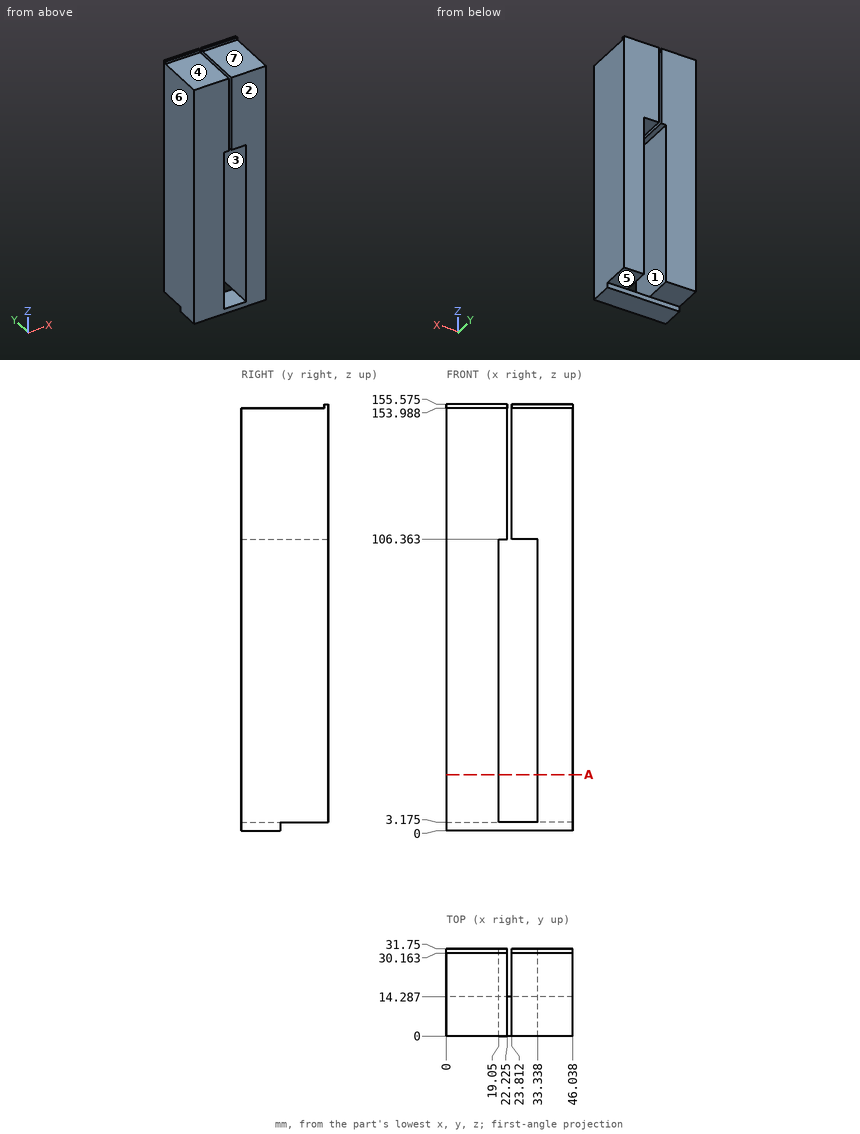
Job drawing, mm, ordinate dimensions from the low corner. One solid piece. A direction names the side the tool comes from. Round coordinates to 2 decimals unless told otherwise and drop trailing zeros. Write each loop counter-clockwise with the first axis right and the second up, starting at its lowest first coordinate (ties: lowest second). Pieces come first, ordered by that corner, then holes. Notation, with made-up numbers: (55, 5.25) -> (88, 5.25) arc R11 ccw to (88, 15.25) -> close; hole circle Ø6 at (76.5, 35). An arc over 180 degrees is marked (long way). Answer as a JSON object with one key per item and string values.
(1) Band-saw the part on A-A, the plane z = 20.5. List the corners of the cut face in (x, y).
Reported:
{"outline": "(0, 0) -> (19.05, 0) -> (19.05, 31.75) -> (0, 31.75) -> close; (33.34, 0) -> (46.04, 0) -> (46.04, 31.75) -> (33.34, 31.75) -> close"}
(2) Pin check, flat tips, straight feed: P1, Ø11, axis at x = 34.5, y = 20, coming from the +Z side; P2, Ø0.5, axis at x = 11, z = 155, coming from the -Y side; P3, Ø1.5, axis at x = 12.5, y = 22.5, coming from the -Z side (1 decimal). Stop position of each tip, or through.
Reported:
{"P1": "stops at z = 153.99", "P2": "stops at y = 30.16", "P3": "stops at z = 3.2"}
(3) Which spindle directions (+Z, -Z, +X, -X, +Y, -Y) get a long thin tool onto all of the face, cutting with end or side? Do the marked faces 5, 6 and 7. Say none if no direction does.
Reported:
{"face 5": "-Z, +X, -X, +Y", "face 6": "+Z, -Z, -X, +Y, -Y", "face 7": "+Z, +X, -X, -Y"}
(4) Probe probe 1 along X at (y, z) = (13, 66.5); probe 2 along Z at (x, y) = (30, 4) (1 decimal); probe 3 along X at (y, z) = (13, 136) (1 decimal). List the from-to ranges inside material, lowest first. Write a range as [from, to].
Reported:
{"probe 1": "x = [0, 19.05], [33.34, 46.04]", "probe 2": "z = [0, 3.2], [106.4, 154]", "probe 3": "x = [0, 22.2], [23.8, 46]"}
(5) Two-plate mould, pull along Z, no slides. Class the marked faces 1, 2, 3 and 4: +Z half, -Z half, draft (parallel to the pull), parting line (faces both ways), or undercut.
Reported:
{"face 1": "undercut", "face 2": "draft", "face 3": "undercut", "face 4": "+Z half"}
